Job drawing, mm, ordinate dimensions from the low corner. One solid piece. Coordinates: 2 decimals unless noted, no trailing zeros. Write each loop counter-clockwise with the first axis right and the second up, starting at its lowest first coordinate (ties: lowest second). Pieces come first, ordered by that corner, then holes. Notation, with made-up numbers: (66, 41.25) - (120, 41.25) arc R15 cw to (120, 51.25) - close; hole circle Ø9 at (44.25, 37). An arc over 180 degrees is marked (long way). Put each result on its own line as item: value. Start each with the question number.
1. Pull direction X, two halves, no side cores. Call the marked faces 1, 2, 3 and 4: released by +X, released by -X, zero draft, split by the parting line, or undercut.
2. Saw through at A-A, the plane x = 7.5. Write the cut outline in (y, z), plus the area to 3 significant figures.
3. Saw through at C-C, the plane y = 6. Write the cut outline in (x, z), plus the area to 3 significant figures.
4. Saw through at D-D, the plane x = 12.5. Write the cut outline in (y, z) (3 decimals), plus the area to 3 significant figures.
5. Saw through at B-B, the plane z = 2.45. Write the cut outline in (x, y).
6. Drill centre lines: L1, parallel to X at y = 5, z = 0.85; L2, parallel to X at y = 5.25, z = 2.65; L3, parallel to Y at x = 13.25, z = 2. Where is each one in solid material? Low to high. Write a range as from..to.
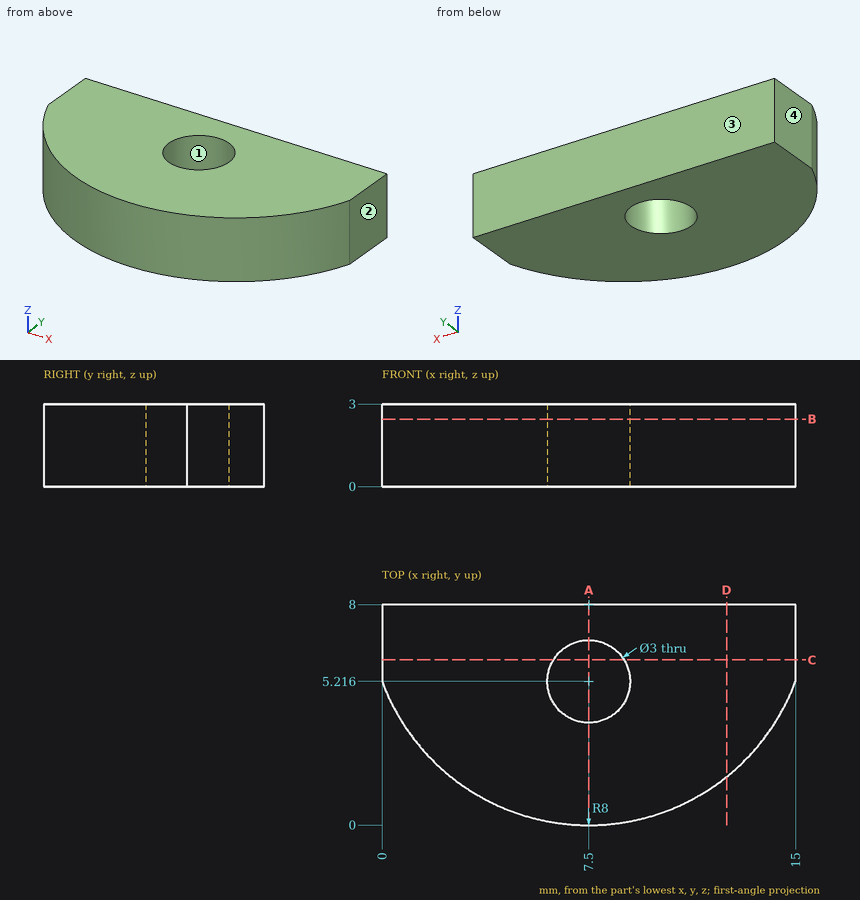
Final values:
1. face 1: undercut
1. face 2: released by +X
1. face 3: zero draft
1. face 4: released by -X
2. outline: (0, 0) - (3.72, 0) - (3.72, 3) - (0, 3) - close; (6.72, 0) - (8, 0) - (8, 3) - (6.72, 3) - close
2. area: 15.0 mm²
3. outline: (0, 0) - (6.22, 0) - (6.22, 3) - (0, 3) - close; (8.78, 0) - (15, 0) - (15, 3) - (8.78, 3) - close
3. area: 37.3 mm²
4. outline: (1.755, 0) - (8, 0) - (8, 3) - (1.755, 3) - close
4. area: 18.7 mm²
5. outline: (0, 5.22) arc R8 ccw to (15, 5.22) - (15, 8) - (0, 8) - close; hole circle Ø3 at (7.5, 5.22)
6. L1: x = 0.08..6.02, 8.98..14.92
6. L2: x = 0..6, 9..15
6. L3: y = 2.44..8
